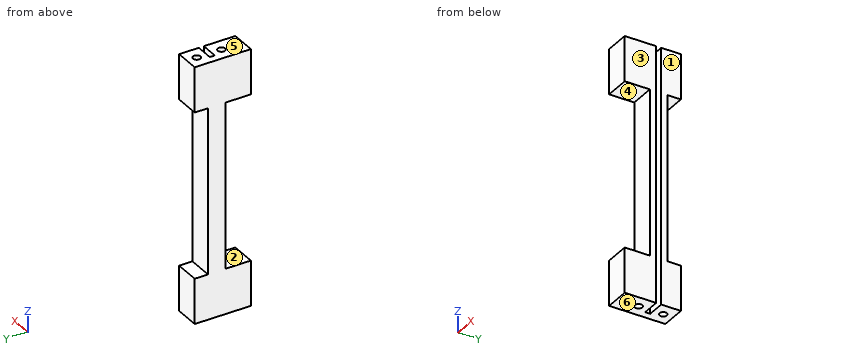
from build123d import *

# Parameters (mm, degrees)
BOSS_EXTRUDE2_DEPTH            = 8.5
SKETCH6_W                      = 6
SKETCH6_H                      = 1.7
CUT_EXTRUDE3_DEPTH             = 87.5
M3X0_5_TAPPED_HOLE4_AT_2_COUNT = 2
M3X0_5_TAPPED_HOLE4_AT_2_PITCH = 8.35
SKETCH20_W                     = 8.5
SKETCH20_H                     = 15.25
BOSS_EXTRUDE3_DEPTH            = 4
SKETCH23_W                     = 8.5
SKETCH23_H                     = 15.25
BOSS_EXTRUDE4_DEPTH            = 4


with BuildPart() as part:
    # Sketch5 → Boss-Extrude2 (new body)
    with BuildSketch(Plane(origin=(0, 0, 0), x_dir=(0, 0, -1), z_dir=(1, 0, 0))):
        Polygon((0, 0), (15.25, 0), (15.25, 4.5), (71.25, 4.5), (71.25, 0), (86.5, 0), (86.5, 15), (71.25, 15), (71.25, 10.5), (15.25, 10.5), (15.25, 15), (0, 15), align=None)
    extrude(amount=BOSS_EXTRUDE2_DEPTH)

    # Sketch6 → Cut-Extrude3 (cut, through all)
    with BuildSketch(Plane.XY):
        with Locations((5.5, 7.5)):
            Rectangle(SKETCH6_W, SKETCH6_H)
    extrude(amount=-CUT_EXTRUDE3_DEPTH, mode=Mode.SUBTRACT)

    # Sketch18 → M3x0.5 Tapped Hole4 (revolve, cut)
    with BuildSketch(Plane(origin=(4.25, 3.325, 0), x_dir=(0, -1, 0), z_dir=(1, 0, 0))):
        Polygon((0, 0), (0, 6.751075774), (1.25, 6), (1.25, 0), align=None)
    m3x0_5_tapped_hole4 = revolve(axis=Axis((4.25, 3.325, 6.35), (0, 0, -1)), mode=Mode.SUBTRACT)

    # M3x0.5 Tapped Hole4 at 2: M3x0.5 Tapped Hole4 ×2
    with Locations(*[(0, i * M3X0_5_TAPPED_HOLE4_AT_2_PITCH, 0) for i in range(1, M3X0_5_TAPPED_HOLE4_AT_2_COUNT)]):
        add(m3x0_5_tapped_hole4, mode=Mode.SUBTRACT)

    # Mirror3: M3x0.5 Tapped Hole4 across plane
    add(m3x0_5_tapped_hole4.mirror(Plane(origin=(0, 0, -43.25), x_dir=(1, 0, 0), z_dir=(0, 0, -1))), mode=Mode.SUBTRACT)

    # Mirror3 copy 1 sketch → Mirror3 copy 1 (revolve, cut)
    with BuildSketch(Plane(origin=(4.25, 11.675, -86.5), x_dir=(0, -1, 0), z_dir=(1, 0, 0))):
        Polygon((0, 0), (0, -6.751075774), (1.25, -6), (1.25, 0), align=None)
    revolve(axis=Axis((4.25, 11.675, -92.85), (0, 0, -1)), mode=Mode.SUBTRACT)

    # Sketch20 → Boss-Extrude3 (add)
    with BuildSketch(Plane.XZ):
        with Locations((4.25, -7.625)):
            Rectangle(SKETCH20_W, SKETCH20_H)
    extrude(amount=BOSS_EXTRUDE3_DEPTH)

    # Sketch23 → Boss-Extrude4 (add)
    with BuildSketch(Plane.XZ):
        with Locations((4.25, -78.875)):
            Rectangle(SKETCH23_W, SKETCH23_H)
    extrude(amount=BOSS_EXTRUDE4_DEPTH)


solid = part.part
The listing builds one solid part. Answer for the finished solid, in the listing's coordinates (mm). Face numbers are marked on the shaded views. A direction names the side the tool comes from. Coordinates: 2 decimals unless noted, no trailing zeros. Write each loop counter-clockwise with the first axis right and the second up, starting at its lowest first coordinate (ties: lowest second). Pieces come first, ordered by that corner, then holes. Notation, with made-up numbers: (24, -32) - (57, -32) arc R22 ccw to (57, -3) - close; hole circle Ø8 at (80, 59). An arc over 180 degrees is marked (long way). Put each result on its own line as item: value.
1. The part is cut by section C-C on z = -14. Give the vertices of the cut face in (x, y), plus the area to 3 significant figures.
Answer sheet:
outline: (0, -4) - (8.5, -4) - (8.5, 6.65) - (2.5, 6.65) - (2.5, 8.35) - (8.5, 8.35) - (8.5, 15) - (0, 15) - close
area: 151 mm^2
2. A tool of negligible diameter and unlimited length cuts with its end or side. For the marked faces 1 and 2, from which of +Z, -Z, +X, -X, +Y, -Y can it reach the whole face along a straight path? Write none if from no direction.
Answer sheet:
face 1: +Z, -Z, +X, +Y, -Y
face 2: +X, -X, -Y
3. Find the intervals of material crossed by line 1 along Y through (x, z) = (4.25, -1.75) (3 decimals); line 2 along Y through (x, z) = (6.25, -70); line 3 along Y through (x, z) = (3, -9.5), in increasing order. Write a range as from..to.
Answer sheet:
line 1: y = -4..2.075, 4.575..6.65, 8.35..10.425, 12.925..15
line 2: y = 4.5..6.65, 8.35..10.5
line 3: y = -4..6.65, 8.35..15
4. The part is cut by section B-B on x = 7.5. Give the vertices of the cut face in (y, z).
Answer sheet:
outline: (-4, -86.5) - (6.65, -86.5) - (6.65, 0) - (-4, 0) - (-4, -15.25) - (4.5, -15.25) - (4.5, -71.25) - (-4, -71.25) - close; (8.35, -86.5) - (15, -86.5) - (15, -71.25) - (10.5, -71.25) - (10.5, -15.25) - (15, -15.25) - (15, 0) - (8.35, 0) - close
5. The part is cut by section D-D on z = -41. Give the vertices of the cut face in (x, y).
Answer sheet:
outline: (0, 4.5) - (8.5, 4.5) - (8.5, 6.65) - (2.5, 6.65) - (2.5, 8.35) - (8.5, 8.35) - (8.5, 10.5) - (0, 10.5) - close
6. Flat-ended cylindrical pins translate along their axes: pin 1 Ø4 at (x, y) = (4, -0.5) entering from +Z; pin 2 Ø4 at (x, z) = (2.5, -29.5) entering from +Y; pin 3 Ø1 at (y, z) = (12.5, -69.5) entering from -X; pin 4 Ø2 at (x, y) = (4.25, 3.325) entering from +Z. Find the tip coordinate at first contact, or state that the pin passes through.
Answer sheet:
pin 1: stops at z = 0
pin 2: stops at y = 10.5
pin 3: passes through
pin 4: stops at z = -6.15
7. The part is cut by section A-A on y = -2. Give the vertices of the cut face in (x, z).
Answer sheet:
outline: (0, -86.5) - (8.5, -86.5) - (8.5, -71.25) - (0, -71.25) - close; (0, -15.25) - (8.5, -15.25) - (8.5, 0) - (0, 0) - close
8. Determine the mould class of the marked faces 3, 4, 5 and 6 for opening direction Z: pulls with the +Z half, pulls with the -Z half, needs draft (parallel to the pull), parting line crosses it, or undercut.
Answer sheet:
face 3: needs draft
face 4: undercut
face 5: pulls with the +Z half
face 6: pulls with the -Z half
